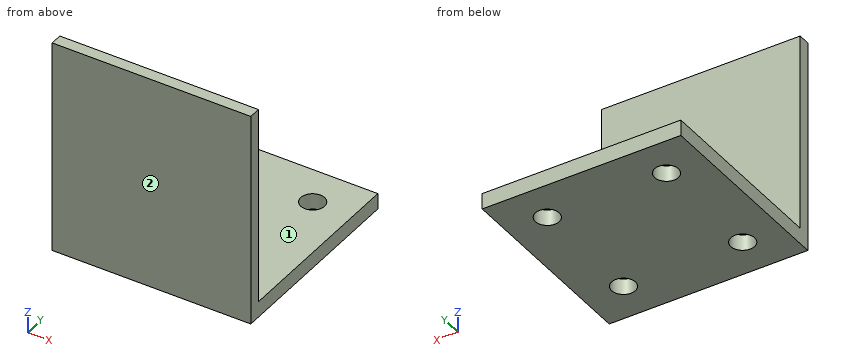
```python
from build123d import *

# Parameters (mm, degrees)
F0_W     = 50
F0_H     = 50
F1_DEPTH = 4
F2_W     = 50
F2_H     = 3
F3_DEPTH = 50
F4_R     = 3
F5_DEPTH = 25


with BuildPart() as f1:
    # F0 (on Top) → F1 (new body)
    with BuildSketch(Plane.XY):
        Rectangle(F0_W, F0_H)
    extrude(amount=F1_DEPTH)

    # F2 (on face) → F3 (join)
    with BuildSketch(Plane.XY.offset(4)):
        with Locations((0, -23.5)):
            Rectangle(F2_W, F2_H)
    extrude(amount=F3_DEPTH)

    # F4 (on face) → F5 (cut)
    with BuildSketch(Plane.XY.offset(4)):
        with Locations((-15, 15)):
            Circle(F4_R)
        with Locations((-15, -15)):
            Circle(F4_R)
        with Locations((15, -15)):
            Circle(F4_R)
        with Locations((15, 15)):
            Circle(F4_R)
    extrude(amount=-F5_DEPTH, mode=Mode.SUBTRACT)


solid = f1.part
```
Here's how the part is built. I have some questions about the finished solid (model axes, mm). Face numbers are marked on the shaded views. A direction names the side the tool comes from. Round coordinates to 2 decimals unless told otherwise and drop trailing zeros. Order: outer loops, then holes, each group sorted by start corner. A loop starts at its lowest first (then second) coordinate and runs counter-clockwise, first axis right, second up. Notation, with made-up numbers: (81, 34.5) -> (131, 34.5) arc R25 ccw to (131, 56.5) -> close; hole circle Ø10 at (22, -16). An arc over 180 degrees is marked (long way). Use a Markdown table: item, result. Add a question column.
(1) Suppose I cut it at A-A, the plane y = 15. Please give me the cut outline in (x, z).
(2) Suppose I cut it at B-B, the plane x = 15. Please give me the cut outline in (y, z).
(3) Suppose I cut it at D-D, the plane y = -13.5. Please give me the cut outline in (x, z), and give its area (3 significant figures).
(4) Suppose I cut it at C-C, the plane x = 21.5. Please give me the cut outline in (y, z).
(5) I need wall thicknesses on line 1 along Y through (x, z) = (15, 2); line 2 along Y through (x, z) = (-16, 19); line 3 along Z through (x, y) = (7.5, 0). Which ranges of each line are inside material? Lowest first, please.
(6) For the marked faces 1 and 2, which set-ups out of +Z, -Z, +X, -X, +Y, -Y let a thin tool reach every point of the face, with its end or its side?
(7) For pin 1 Ø5 at (x, z) = (-14.5, 47.5) entering from +Y; pin 2 Ø8 at (x, y) = (-15, -15) entering from -Z; pin 3 Ø7 at (x, y) = (15, -15) entering from +Z; pin 4 Ø3.5 at (x, y) = (-15, 15) entering from -Z, each with a flat end and sliding along its axis, tell me the tip position at first contact or that it passes through.
Verdict:
| question | item | result |
|---|---|---|
| 1 | outline | (-25, 0) -> (-18, 0) -> (-18, 4) -> (-25, 4) -> close; (-12, 0) -> (12, 0) -> (12, 4) -> (-12, 4) -> close; (18, 0) -> (25, 0) -> (25, 4) -> (18, 4) -> close |
| 2 | outline | (-25, 0) -> (-18, 0) -> (-18, 4) -> (-22, 4) -> (-22, 54) -> (-25, 54) -> close; (-12, 0) -> (12, 0) -> (12, 4) -> (-12, 4) -> close; (18, 0) -> (25, 0) -> (25, 4) -> (18, 4) -> close |
| 3 | outline | (-25, 0) -> (-17.6, 0) -> (-17.6, 4) -> (-25, 4) -> close; (-12.4, 0) -> (12.4, 0) -> (12.4, 4) -> (-12.4, 4) -> close; (17.6, 0) -> (25, 0) -> (25, 4) -> (17.6, 4) -> close |
| 3 | area | 158 mm2 |
| 4 | outline | (-25, 0) -> (25, 0) -> (25, 4) -> (-22, 4) -> (-22, 54) -> (-25, 54) -> close |
| 5 | line 1 | -25 to -18, -12 to 12, 18 to 25 |
| 5 | line 2 | -25 to -22 |
| 5 | line 3 | 0 to 4 |
| 6 | face 1 | +Z, +X, -X, +Y |
| 6 | face 2 | +Z, -Z, +X, -X, -Y |
| 7 | pin 1 | y = -22 |
| 7 | pin 2 | z = 0 |
| 7 | pin 3 | z = 4 |
| 7 | pin 4 | through |
